Read the model definition and answer for the solid it produces. Units are mm, in the model's axes. A direction names the side the tool comes from. Give positions to 0.01 mm unless a question says otherwise; leave off trailing zeros. Write each loop counter-clockwise with the first axis right and the second up, starting at its lowest first coordinate (ties: lowest second). Pieces come first, ordered by that corner, then holes.
```python
from build123d import *

# Parameters (mm, degrees)
BOSS_EXTRUDE1_DEPTH = 19.05
CUT_EXTRUDE1_DEPTH  = 311.977162881


with BuildPart() as part:
    # Sketch1 → Boss-Extrude1 (new body)
    with BuildSketch(Plane(origin=(0, 0, 0), x_dir=(1, 0, 0), z_dir=(0, 1, 0))):
        Polygon((-234.635149399, 0), (-117.317574699, -203.2), (117.317574699, -203.2), (234.635149399, 0), (117.317574699, 203.2), (-117.317574699, 203.2), align=None)
    extrude(amount=BOSS_EXTRUDE1_DEPTH)

    # Sketch2 → Cut-Extrude1 (cut, through all)
    with BuildSketch(Plane(origin=(0, 19.05, 0), x_dir=(1, 0, 0), z_dir=(0, 1, 0))):
        with BuildLine():
            Line((-29.972, -155.702), (29.972, -155.702))
            ThreePointArc((29.972, -155.702), (40.005, -165.735), (29.972, -175.768))
            Line((29.972, -175.768), (-29.972, -175.768))
            ThreePointArc((-29.972, -175.768), (-40.005, -165.735), (-29.972, -155.702))
        make_face()
        with BuildLine():
            Line((-119.85588742, 103.807513402), (-149.82788742, 51.894486598))
            ThreePointArc((-149.82788742, 51.894486598), (-163.533220296, 48.222153722), (-167.205553172, 61.927486598))
            Line((-167.205553172, 61.927486598), (-137.233553172, 113.840513402))
            ThreePointArc((-137.233553172, 113.840513402), (-123.528220296, 117.512846278), (-119.85588742, 103.807513402))
        make_face()
        with BuildLine():
            Line((149.82788742, 51.894486598), (119.85588742, 103.807513402))
            ThreePointArc((119.85588742, 103.807513402), (123.528220296, 117.512846278), (137.233553172, 113.840513402))
            Line((137.233553172, 113.840513402), (167.205553172, 61.927486598))
            ThreePointArc((167.205553172, 61.927486598), (163.533220296, 48.222153722), (149.82788742, 51.894486598))
        make_face()
    extrude(amount=-CUT_EXTRUDE1_DEPTH, mode=Mode.SUBTRACT)


solid = part.part
```
Item 1: Determine the mould class of faces 1 (the flat face through (-3, 0, -3)), 2 (the flat face through (175.155, 9.392, 103.022)), 3 (the flat face through (-152.43, 9.66, -87.52)), 4 (the cylindrical face through (123.34, 9.66, -117.4)) for opening direction Z: pulls with the +Z half, pulls with the -Z half, needs draft (parallel to the pull), parting line crosses it, or undercut.
Result set:
face 1: needs draft
face 2: pulls with the +Z half
face 3: undercut
face 4: undercut
Item 2: Section B-B (z = 161) is taken. Write down the section's boundary in (x, y), and give its area (3 significant figures).
Result set:
outline: (-141.68, 0) - (-38.82, 0) - (-38.82, 19.05) - (-141.68, 19.05) - close; (38.82, 0) - (141.68, 0) - (141.68, 19.05) - (38.82, 19.05) - close
area: 3,920 mm2
Item 3: Which of the six approach directions +Z, -Z, +X, -X, +Y, -Y give full straight-line access (tool end or side, diameter ignored) to faces 5 (the flat face through (176.798, 9.392, -100.178)), 6 (the cylindrical face through (-40, 10, 166))?
Result set:
face 5: -Z, +X, +Y, -Y
face 6: +Y, -Y
Item 4: Section C-C (x = -175) is taken. Write down the section's boundary in (y, z), and give its area (3 significant figures).
Result set:
outline: (0, -103.29) - (19.05, -103.29) - (19.05, 103.29) - (0, 103.29) - close
area: 3,940 mm2
Item 5: Section A-A (y = 16) is taken. Write down the section's boundary in (x, z) (3 decimals), and give its area (3 significant figures).
Result set:
outline: (-234.635, 0) - (-117.318, -203.2) - (117.318, -203.2) - (234.635, 0) - (117.318, 203.2) - (-117.318, 203.2) - close; hole (-167.206, -61.927) - (-137.234, -113.841) arc R10.033 ccw to (-119.856, -103.808) - (-149.828, -51.894) arc R10.033 ccw to start; hole (-29.972, 155.702) - (29.972, 155.702) arc R10.033 ccw to (29.972, 175.768) - (-29.972, 175.768) arc R10.033 ccw to start; hole (119.856, -103.808) arc R10.033 ccw to (137.234, -113.841) - (167.206, -61.927) arc R10.033 ccw to (149.828, -51.894) - close
area: 138,000 mm2
Item 6: Section D-D (z = -175.5) is taken. Write down the section's boundary in (x, y), and give its area (3 significant figures).
Result set:
outline: (-133.31, 0) - (133.31, 0) - (133.31, 19.05) - (-133.31, 19.05) - close
area: 5,080 mm2
Item 7: Each of these flat-tipped pins is pushed along its axis until it touches: pin 1 Ø2 at (x, y) = (143, 4) entering from -Z; pin 2 Ø1.5 at (x, y) = (-166, 7) entering from -Z; pin 3 Ø1 at (x, y) = (120, 13.5) entering from +Z. Where does it stop, or does it pass through?
Result set:
pin 1: stops at z = -160.45
pin 2: stops at z = -120.18
pin 3: stops at z = 199.42
Item 8: Find the intervals of material crossed by line 1 along Z through (x, y) = (0, 2); line 2 along X through (y, z) = (8.75, -78); line 3 along Z through (x, y) = (127.5, 3), in increasing order.
Result set:
line 1: z = -203.2 to 155.7, 175.77 to 203.2
line 2: x = -189.6 to -157.93, -134.76 to 134.76, 157.93 to 189.6
line 3: z = -185.56 to -118.8, -90.57 to 185.56
